Autodesk Inventor part; units mm, degrees
ref_plane "Start Plane" through (-5.7625, 0, 0) normal (1, 0, 0) x (0, 1, 0)
ref_plane "End Plane" through (15.7875, 0, 0) normal (1, 0, 0) x (0, 1, 0)
ref_plane "Loft Start Plane" through (0, 0, 7) normal (0, 0, 1) x (1, 0, 0)
ref_plane "Start Plane" through (-5.7625, 0, 0) normal (1, 0, 0) x (0, 1, 0)
ref_plane "End Plane" through (15.7875, 0, 0) normal (1, 0, 0) x (0, 1, 0)
sketch "Box Sketch" plane through (0, 0, 0) normal (1, 0, 0) x (0, 1, 0)
  line L0 (-3.9688, 0) -> (3.9688, 0)
  line L1 (3.9688, 0) -> (3.9688, 10)
  line L2 (3.9688, 10) -> (-3.9688, 10)
  line L3 (-3.9688, 10) -> (-3.9688, 0)
  line L4 (-1.9688, 2) -> (1.9688, 2)
  line L5 (1.9688, 2) -> (1.9687, 7)
  line L6 (1.9687, 7) -> (-1.9687, 7)
  line L7 (-1.9687, 7) -> (-1.9688, 2)
  line L8 (1.9688, 2) -> (3.9688, 2) construction
  line L9 (-1.9688, 2) -> (-3.9688, 2) construction
  line L10 (-1.9688, 2) -> (-1.9688, 0) construction
  line L11 (2.7188, 1.25) -> (2.7188, 7.75)
  line L12 (2.7188, 7.75) -> (-2.7188, 7.75)
  line L13 (-2.7188, 7.75) -> (-2.7188, 1.25)
  line L14 (-2.7188, 1.25) -> (2.7188, 1.25)
  line L15 (-1.9687, 7) -> (-2.7188, 7) construction
  line L16 (1.9687, 7) -> (2.7188, 7) construction
  line L17 (1.9688, 2) -> (1.9687, 1.25) construction
  line L18 (-1.9687, 7) -> (-1.9687, 7.75) construction
  line L19 (-2.8688, 7.9) -> (2.8688, 7.9)
  line L20 (2.8688, 7.9) -> (2.8688, 1.1)
  line L21 (2.8688, 1.1) -> (-2.8688, 1.1)
  line L22 (-2.8688, 1.1) -> (-2.8688, 7.9)
  point P0 (0, 0)
  point P1 (0, 0)
  dimension "boxHeight" = 7.9375
  dimension "boxWidth" = 10
  dimension "frontWallThick" = 3
  dimension "sideWallThick" = 2
  dimension "connectorTol" = 0.15
  dimension "d24" = 0.75
sketch "Fitting Sketch" plane through (0, 0, 0) normal (1, 0, 0) x (0, 1, 0)
  line L0 (0, 10) -> (0, 14.5) construction
  line L1 (2.3813, 10) -> (2.3813, 12.0417)
  line L2 (2.3813, 12.0417) -> (3.175, 12.5)
  line L3 (3.175, 12.5) -> (2.3813, 14.5)
  line L4 (2.3813, 14.5) -> (1.5, 14.5)
  line L5 (1.5, 14.5) -> (1.5, 10)
  line L6 (1.5, 10) -> (2.3813, 10)
  point P0 (0, 0)
  dimension "d2" = 3
  dimension "d3" = 2
  dimension "d4" = 60
  dimension "d5" = 2.5
  dimension "d6" = 4.7625
  dimension "d7" = 6.35
  dimension "d9" = 10
revolve "Fitting" add sketch "Fitting Sketch" angle 360 about axis through (0, 0, 10) along (0, 0, 1)
extrude "Box" add sketch "Box Sketch" along normal mid plane 11.525 contours L3 L2 L1 L0 | L14 L13 L12 L11 | L19 L20 L21 L22
ref_plane "Loft Start Plane" through (0, 0, 7) normal (0, 0, 1) x (1, 0, 0)
sketch "Loft Sketch" plane through (0, 0, 7) normal (0, 0, 1) x (1, 0, 0)
  line L0 (1.5, -1.9688) -> (-1.5, -1.9688)
  line L1 (-1.5, -1.9688) -> (-1.5, 1.9687)
  line L2 (-1.5, 1.9687) -> (1.5, 1.9687)
  line L3 (1.5, 1.9687) -> (1.5, -1.9688)
  line L4 (1.5, -1.9688) -> (-1.5, 1.9687) construction
  line L5 (-1.5, -1.9688) -> (1.5, 1.9687) construction
  point P0 (0, 0)
  dimension "d17" = 3
  dimension "d18" = 3.9375
loft "Loft" cut profiles "Loft Sketch" section 1 edges at (0, -1.5, 10)
pattern_linear "Channel Repetition" count 2 spacing 10.775 along (1, 0, 0)
extrude "Clip Extra Length" cut sketch "Box Sketch" along normal blind 19.45 from surface at 15.7875 contours L3 L2 L1 L0 | L19 L20 L21 L22
extrude "Connector" add sketch "Box Sketch" along normal blind 3.6625 from surface at 15.7875 contours L14 L13 L12 L11
equation "\"boxHeight\" = fittingBarbOD + 2 * siliconeThick"
equation "\"boxWidth\" = manifoldWidth"
equation "\"d2\" = fittingID"
equation "\"d3\" = fittingBarbLength"
equation "\"d4\" = fittingBarbBaseAngle"
equation "\"d5\" = fittingNeckLength"
equation "\"d6\" = fittingOD"
equation "\"d7\" = fittingBarbOD"
equation "\"d14\" = blockWidth"
equation "\"d27\" = chanWidth"
equation "\"d17\" = fittingID"
equation "\"d18\" = boxHeight - 2 * sideWallThick"
equation "\"d16\" = boxWidth - frontWallThick"
equation "\"d29\" = -0.5 * blockWidth"
properties part number "manifold_lower" material "PLA (Blue-glowing, 3D Printed)"
Can you work these out from the model? Positions are in its coordinate system, mm. A direction names the side the tool comes from. Coordinates: 2 decimals unless noted, no trailing zeros. Order: outer loops, then holes, each group sorted by start corner. A loop starts at its lowest first (then second) coordinate and runs counter-clockwise, first axis right, second up.
1. I need wall thicknesses on line 1 (X direction, y = 0, z = 11.45) (3 decimals); line 2 (Y direction, x = -0.75, z = 2.75); line 3 (Z direction, x = 5, y = 1.25). Which ranges of each line are inside material? Lowest first, please.
2. If we section it at C-C (y = 0): Give the number of separate pieces and of enclosed holes in the cut face, then the cut area to 3 significant figures.
3. Thinking about a two-plate mould opening in Z: for faces 1 (the face through (11, 2, 14.5)), 2 (the face through (8.767, 1.28, 11.035)), 3 (the face through (18, -2.719, 5)), which applies, +Z half, -Z half, draft (parallel to the pull), parting line (faces both ways), or undercut?
4. For faces 4 (the face through (18, 0, 1.25)), 5 (the face through (2.11, 1.1, 11.04)), 6 (the face through (0.07, -1.5, 12.22)), 7 (the face through (2, 0, 14.5)), 8 (the face through (7, 0, 2)), which set-ups out of +Z, -Z, +X, -X, +Y, -Y let a thin tool reach every point of the face, with its end or its side?
5. If we section it at B-B (z = 6.25): Please give me the cut outline in (x, y).
6. If we section it at A-A (x = 17.5): Please give me the cut outline in (y, z).
7. I'm going to push flat-ended pins straight in: pin 1 (1.8 mm diameter, centred on x = 18.5, z = 4, fed in from +Y); pin 2 (1.1 mm diameter, centred on x = 17, y = 0.5, fed in from +Z); pin 3 (1.8 mm diameter, centred on x = 18.5, z = 3.5, fed in from -Y). Where does each tip first touch, or does it pass through?
Entries:
1. line 1: x = -2.381 to -1.5, 1.5 to 2.381, 8.394 to 9.275, 12.275 to 13.156
1. line 2: y = -3.97 to -1.97, 1.97 to 3.97
1. line 3: z = 0 to 2, 7 to 10
2. separate pieces: 4
2. enclosed holes: 0
2. area: 115 mm2
3. face 1: +Z half
3. face 2: undercut
3. face 3: draft
4. face 4: -Z, +X, +Y, -Y
4. face 5: none
4. face 6: +Z
4. face 7: +Z, +X, -X, +Y, -Y
4. face 8: +X, -X
5. outline: (-5.76, -3.97) - (15.79, -3.97) - (15.79, -2.72) - (19.45, -2.72) - (19.45, -1.97) - (-5.76, -1.97) - close; (-5.76, 1.97) - (19.45, 1.97) - (19.45, 2.72) - (15.79, 2.72) - (15.79, 3.97) - (-5.76, 3.97) - close
6. outline: (-2.72, 1.25) - (2.72, 1.25) - (2.72, 7.75) - (-2.72, 7.75) - close; hole (-1.97, 2) - (1.97, 2) - (1.97, 7) - (-1.97, 7) - close
7. pin 1: stops at y = 2.72
7. pin 2: stops at z = 7.75
7. pin 3: stops at y = -2.72
